Geometry: final body of the model. Coordinates: model frame, mm. Face numbers are marked on the shaded views. Round coordinates to 2 decimals unless told otherwise and drop trailing zeros. Order: outer loops, then holes, each group sorted by start corner. A loop starts at its lowest first (then second) coordinate and runs counter-clockwise, first axis right, second up. Notation, with made-up numbers: M 57,30.25 L 82,30.25 A8 cw 82,42.25 Z; hole C 39.5,53 d7. An arc over 180 degrees is marked long. Put each result on its own line as item: value. Start each with the question number.
1) Section B-B, the plane x = 18. Return loops of the section in (y, z).
2) Section C-C, the plane z = 197. Return loops of the section in (x, y) (3 decimals).
3) Material intervals for probe 1 along X at (y, z) = (18.75, 184); probe 2 along Y at (x, z) = (7, 205.5); probe 3 along X at (y, z) = (2.5, 130), sorted ascending. Write a range as [from, to].
4) Section A-A, the plane y = 6.5. Return loops of the section in (x, z).
5) First-contact query: P1, Ø10, axis at x = 18.5, y = 6.5, coming from the -Z side. Flat tip, straight axial feed; report the tip coordinate or a pass-through.
6) Draft query along X for the marked faces 1 and 2. Return one class per face: pulls with the +X half, pulls with the -X half, needs draft (parallel to the pull), parting line crosses it, or undercut.
Autodesk Inventor part; units mm, degrees
ref_plane "YZ Plane" through (0, 0, 0) normal (1, 0, 0) x (0, 1, 0)
ref_plane "XZ Plane" through (0, 0, 0) normal (0, 1, 0) x (-1, 0, 0)
ref_plane "XY Plane" through (0, 0, 0) normal (0, 0, 1) x (1, 0, 0)
sketch "Sketch1" plane through (0, 0, 0) normal (0, 0, 1) x (1, 0, 0)
  line L0 (3.7363, 0) -> (22.7863, 0)
  line L1 (25.9613, 3.175) -> (25.9613, 22.225)
  line L2 (22.7863, 25.4) -> (3.7363, 25.4)
  line L3 (0.5613, 22.225) -> (0.5613, 3.175)
  arc A0 (3.7363, 25.4) -> (0.5613, 22.225) centre (3.7363, 22.225) ccw
  arc A1 (0.5613, 3.175) -> (3.7363, 0) centre (3.7363, 3.175) ccw
  arc A2 (22.7863, 0) -> (25.9613, 3.175) centre (22.7863, 3.175) ccw
  arc A3 (25.9613, 22.225) -> (22.7863, 25.4) centre (22.7863, 22.225) ccw
  line L4 (3.7363, 23.4) -> (22.7863, 23.4)
  arc A4 (23.9613, 22.225) -> (22.7863, 23.4) centre (22.7863, 22.225) ccw
  line L5 (23.9613, 22.225) -> (23.9613, 3.175)
  arc A5 (22.7863, 2) -> (23.9613, 3.175) centre (22.7863, 3.175) ccw
  line L6 (22.7863, 2) -> (3.7363, 2)
  arc A6 (2.5613, 3.175) -> (3.7363, 2) centre (3.7363, 3.175) ccw
  line L7 (2.5613, 3.175) -> (2.5613, 22.225)
  arc A7 (3.7363, 23.4) -> (2.5613, 22.225) centre (3.7363, 22.225) ccw
  point P0 (0, 0)
  point P1 (0.5613, 0)
  point P2 (25.9613, 0)
  point P3 (0.5613, 25.4)
  dimension "d0" = 25.4
  dimension "d2" = 25.4
  dimension "d3" = 3.175
  dimension "d4" = 2
extrude "tube" add sketch "Sketch1" along normal blind 330.1
sketch "Sketch7" plane through (3.7363, 25.4, 0) normal (0, 1, 0) x (1, 0, 0)
  line L0 (19.05, 0) -> (0, 0)
  circle A0 centre (9.525, -25.4) radius 3.5758
  point P0 (-3.7363, 0)
  dimension "d45" = 25.4
hole "centerHole_cutOff" at (13.2613, 25.4, 25.4) direction (0, -1, 0) diameter 6.35 end through all
sketch "Sketch8" plane through (3.7363, 25.4, 0) normal (0, 1, 0) x (1, 0, 0)
  circle A0 centre (9.525, -25.4) radius 3.175
  line L0 (0, 0) -> (0, -330.1)
  circle A1 centre (9.525, -152.4) radius 1.4483
  circle A2 centre (9.525, -302.4) radius 1.4483
  point P0 (-3.7363, 0)
  dimension "d55" = 150
  dimension "d60" = 127
hole "armHoles" at (13.2613, 25.4, 152.4) at (13.2613, 25.4, 302.4) direction (0, -1, 0) diameter 4.5 end through all
sketch "Sketch9" plane through (3.7363, 25.4, 0) normal (0, 1, 0) x (1, 0, 0)
  circle A0 centre (9.525, -25.4) radius 3.175 construction
  line L0 (9.525, -25.4) -> (9.525, -40.0812) construction
  line L1 (-12.1249, -52.4308) -> (9.525, -39.9312)
  line L2 (-8.8213, -52.7845) -> (41.9787, -52.7845) construction
  line L3 (9.525, -40.0812) -> (40.882, -40.0812) construction
  line L4 (9.2652, -40.0812) -> (31.8692, -53.1316)
  line L5 (-12.1249, -52.4308) -> (-12.1249, 11.2848)
  line L6 (31.8692, -53.1316) -> (31.8692, 11.2848)
  line L7 (-12.1249, 11.2848) -> (31.8692, 11.2848)
  point P0 (-3.7363, 0)
  dimension "d68" = 14.6812
  dimension "d70" = 30
extrude "Extrusion4" cut sketch "Sketch9" against normal blind 50.8
properties part number "2f2ax2" material "Steel"
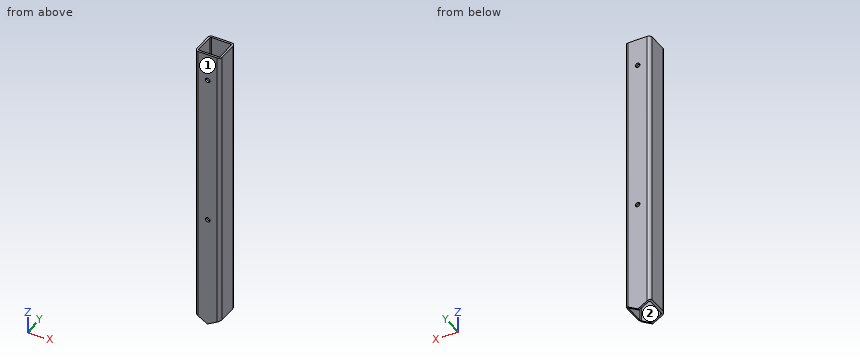
Result sheet:
1. outline: M 0,42.97 L 2,42.97 L 2,330.1 L 0,330.1 Z; M 23.4,42.97 L 25.4,42.97 L 25.4,330.1 L 23.4,330.1 Z
2. outline: M 0.561,3.175 A3.175 ccw 3.736,0 L 22.786,0 A3.175 ccw 25.961,3.175 L 25.961,22.225 A3.175 ccw 22.786,25.4 L 3.736,25.4 A3.175 ccw 0.561,22.225 Z; hole M 2.561,3.175 A1.175 ccw 3.736,2 L 22.786,2 A1.175 ccw 23.961,3.175 L 23.961,22.225 A1.175 ccw 22.786,23.4 L 3.736,23.4 A1.175 ccw 2.561,22.225 Z
3. probe 1: x = [0.56, 2.56], [23.96, 25.96]
3. probe 2: y = [0, 2], [23.4, 25.4]
3. probe 3: x = [0.63, 2.77], [23.75, 25.89]
4. outline: M 0.56,47.26 L 2.56,46.11 L 2.56,330.1 L 0.56,330.1 Z; M 23.96,46.41 L 25.96,47.56 L 25.96,330.1 L 23.96,330.1 Z
5. P1: stops at z = 42
6. face 1: needs draft
6. face 2: undercut
